Can you work these out from the model? Positions are in its coordinate system, mm. Face numbers are marked on the shaded views. A direction names the side the tool comes from. Round coordinates to 2 decimals unless told otherwise and drop trailing zeros. Order: outer loops, then holes, each group sorted by start corner. A loop starts at its lowest first (then second) coordinate and runs counter-clockwise, first axis right, second up.
Q1. We'd pull the mould along Z, two halves only. Please class the marked faces 1, 2 and 3: pulls with the +Z half, pulls with the -Z half, needs draft (parallel to the pull), parting line crosses it, or undercut.
Q2. If I drill on line 1 (X direction, y = 0.15, z = 0); line 2 (X direction, y = -0.7, z = 0); line 3 (Z direction, x = 7, y = -2.25), over which ranges is the centre line in solid material (lowest first)?
Q3. If we section it at A-A (x = 0): Please give me the cut outline in (y, z).
Q4. If we section it at C-C (y = 0.25): Please give me the cut outline in (x, z), plus the area to 3 significant figures.
Q5. If we section it at B-B (z = 0): Please give me the cut outline in (x, y).
Q6. For the marked faces 4 and 5, which set-ups out of +Z, -Z, +X, -X, +Y, -Y let a thin tool reach every point of the face, with its end or its side?
Q7. Will these pins go through, and if not, where does the flat tip stop? P1, Ø1.6, axis at y = 0.5, z = -3, coming from the -X side; P2, Ø3.5, axis at y = 1.5, z = -1, coming from the +X side; P3, Ø0.7, axis at x = 13, z = 1.5, coming from the +Y side; P4, Ø15.5, axis at x = 0, z = 0, coming from the +Y side.
from build123d import *

# Parameters (mm, degrees)
SKETCH1_R           = 14.24
SKETCH1_R_2         = 9.7155
BOSS_EXTRUDE1_DEPTH = 2.794
SKETCH2_W           = 4.55251892
SKETCH2_H           = 21.070507922
CUT_EXTRUDE1_DEPTH  = 3.1242
SKETCH3_R           = 0.75565


with BuildPart() as part:
    # Sketch1 → Boss-Extrude1 (new, symmetric)
    with BuildSketch(Plane(origin=(0, 0, 0), x_dir=(1, 0, 0), z_dir=(0, 1, 0))):
        with Locations(Location((0, 0, 0), (0, 0, 270))):
            Circle(SKETCH1_R)
        with Locations(Location((0, 0, 0), (0, 0, 270))):
            Circle(SKETCH1_R_2, mode=Mode.SUBTRACT)
    extrude(amount=BOSS_EXTRUDE1_DEPTH, both=True)

    # Sketch2 → Cut-Extrude1 (cut)
    with BuildSketch(Plane(origin=(0, 2.794, 0), x_dir=(1, 0, 0), z_dir=(0, 1, 0))):
        with Locations((14.16345946, 0)):
            Rectangle(SKETCH2_W, SKETCH2_H)
    cut_extrude1 = extrude(amount=-CUT_EXTRUDE1_DEPTH, mode=Mode.SUBTRACT)

    # Mirror1: Cut-Extrude1 across plane
    add(cut_extrude1.mirror(Plane(origin=(0, 0, 0), x_dir=(0, 0, 1), z_dir=(1, 0, 0))), mode=Mode.SUBTRACT)

    # Sketch3 → Revolve1 (revolve)
    with BuildSketch(Plane(origin=(0, 0, 0), x_dir=(0, 0, -1), z_dir=(1, 0, 0)), mode=Mode.PRIVATE) as revolve1_sk:
        with Locations((-12.208, -2.794)):
            Circle(SKETCH3_R)
    revolve(revolve1_sk.sketch.rotate(Axis((0, 0, 0), (0, 1, 0)), 236.592446153), axis=Axis((0, 0, 0), (0, 1, 0)))


solid = part.part
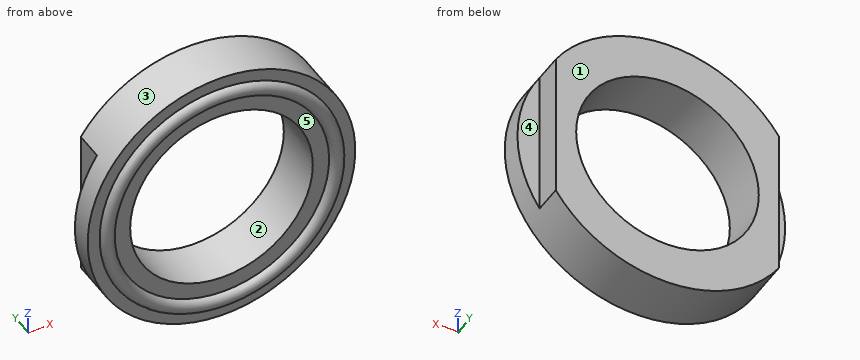
Solution:
1. face 1: needs draft
1. face 2: undercut
1. face 3: parting line crosses it
2. line 1: x = -11.89 to -9.72, 9.72 to 11.89
2. line 2: x = -14.24 to -9.72, 9.72 to 14.24
2. line 3: z = -12.4 to -6.74, 6.74 to 12.4
3. outline: (-2.79, -14.24) - (2.79, -14.24) - (2.79, -9.72) - (-2.79, -9.72) - (-2.79, -11.45) arc R0.76 ccw to (-2.79, -12.96) - close; (-2.79, 9.72) - (2.79, 9.72) - (2.79, 14.24) - (-2.79, 14.24) - (-2.79, 12.96) arc R0.76 ccw to (-2.79, 11.45) - close
4. outline: (-11.89, -7.84) arc R14.24 ccw to (11.89, -7.84) - (11.89, 7.84) arc R14.24 ccw to (-11.89, 7.84) - close; hole circle Ø19.43 at (0, 0)
4. area: 290 mm2
5. outline: (-14.24, -2.79) - (-12.96, -2.79) arc R0.76 ccw to (-11.45, -2.79) - (-9.72, -2.79) - (-9.72, 2.79) - (-11.89, 2.79) - (-11.89, -0.33) - (-14.24, -0.33) - close; (9.72, -2.79) - (11.45, -2.79) arc R0.76 ccw to (12.96, -2.79) - (14.24, -2.79) - (14.24, -0.33) - (11.89, -0.33) - (11.89, 2.79) - (9.72, 2.79) - close
6. face 4: +Z, -Z, +X, +Y
6. face 5: -Y
7. P1: stops at x = -11.89
7. P2: stops at x = 11.89
7. P3: stops at y = -0.33
7. P4: passes through
